Geometry: final body of the model. Coordinates: model frame, mm. Round coordinates to 2 decimals unless told otherwise and drop trailing zeros. Loops run counter-clockwise (first coordinate to the right, second up) from the corner with the lowest first, then second, coordinate; pieces in that order, holes last. Notation, with made-up numbers: M 5,29 L 58,29 A23 cw 58,40 Z; hole C 43.25,74.25 d3. An arc over 180 degrees is marked long. Answer as a JSON object with one key per item and string values.
from build123d import *

# Parameters (mm, degrees)
SKETCH1_R                   = 4.7625
BOSS_EXTRUDE1_DEPTH         = 12.7
FILLET1_R                   = 2.54
F_10_24_TAPPED_HOLE1_REACH  = 41.709
F_10_24_TAPPED_HOLE1_BORE_R = 1.89865


with BuildPart() as part:
    # Sketch1 → Boss-Extrude1 (new body)
    with BuildSketch(Plane.XY):
        with BuildLine():
            Line((-5.46431709, -20.393109008), (0, -11.1125))
            ThreePointArc((0, -11.1125), (11.017431022, -1.450472311), (2.876126639, 10.733850745))
            Line((2.876126639, 10.733850745), (0, 21.1125))
            ThreePointArc((0, 21.1125), (-20.931879636, 2.755734233), (-5.46431709, -20.393109008))
        make_face()
        Circle(SKETCH1_R, mode=Mode.SUBTRACT)
    extrude(amount=BOSS_EXTRUDE1_DEPTH)

    # Fillet1
    fillet1_edges = [part.edges().sort_by_distance(p)[0] for p in [
        (2.876126639, 10.733850745, 6.35),
        (0, -11.1125, 6.35),
        (-5.46431709, -20.393109008, 6.35),
        (0, 21.1125, 6.35),
    ]]
    fillet(fillet1_edges, radius=FILLET1_R)

    # #10-24 Tapped Hole1 bore (on position points) → #10-24 Tapped Hole1 (cut, up to next)
    with BuildSketch(Plane(origin=(11.019222387, -1.436799975, 6.35), x_dir=(0.129295835761, 0.99160606435, 0), z_dir=(0.99160606435, -0.129295835761, 0)), mode=Mode.PRIVATE) as f_10_24_tapped_hole1_sk1:
        with Locations((1e-09, 0)):
            Circle(F_10_24_TAPPED_HOLE1_BORE_R)
    f_10_24_tapped_hole1_tool1 = extrude(f_10_24_tapped_hole1_sk1.sketch, amount=-F_10_24_TAPPED_HOLE1_REACH, mode=Mode.PRIVATE) & part.part
    add(f_10_24_tapped_hole1_tool1.solids().sort_by_distance((11.019222, -1.4368, 6.35))[0], mode=Mode.SUBTRACT)


solid = part.part
1) Ray query, line 1 (Y direction, x = -1, z = 11.5); line 2 (X direction, y = 3.5, z = 4); line 3 (Y direction, x = 0, z = 9.75). Return the intervals inside material, ascending.
Results:
{"line 1": "-12.81 to -4.66, 4.66 to 20.85", "line 2": "-20.82 to -3.23, 3.23 to 10.55", "line 3": "-11.52 to -4.76, 4.76 to 20.15"}
2) Section query B-B (x = 0). Return the cut outline in (y, z).
Results:
{"outline": "M -11.52,0 L -4.76,0 L -4.76,12.7 L -11.52,12.7 Z; M 4.76,0 L 20.15,0 L 20.15,12.7 L 4.76,12.7 Z"}
3) Section query C-C (y = -1). Count the separate pieces of the cut face and the enclosed holes in it, and give its area (3 significant figures).
Results:
{"separate pieces": "3", "enclosed holes": "0", "area": "266 mm2"}
4) Section query D-D (x = -9). Return the cut outline in (y, z).
Results:
{"outline": "M -19.1,0 L 19.1,0 L 19.1,12.7 L -19.1,12.7 Z"}
5) Pull-direction query (Z, two-part tool) for faces 1 (the flat face through (-5, 1, 0)), 2 (the cylindrical face through (7.669, -1.415, 4.496)), 3 (the flat face through (-5, 1, 12.7)), 4 (the flat face through (-2.59, -15.51, 6.26)); classes: +Z half, -Z half, draft (parallel to the pull), parting line (faces both ways), or undercut.
Results:
{"face 1": "-Z half", "face 2": "undercut", "face 3": "+Z half", "face 4": "draft"}
6) Pin query (flat end, axial travel): P1, Ø1, axis at x = -2, y = -12.5, coming from the -Z side; P2, Ø2, axis at y = 17, z = 11, coming from the +X side; P3, Ø5, axis at y = 15, z = 6, coming from the -X side; P4, Ø1, axis at x = 0.5, z = 4.5, coming from the -Y side. Return the tip coordinate at first contact, or that it passes through.
Results:
{"P1": "z = 0", "P2": "x = 1.42", "P3": "x = -17.01", "P4": "y = -11.52"}
7) Section query A-A (z = 11.75). Return the cut outline in (x, y) (1 decimal).
Results:
{"outline": "M -7.5,-19.7 A2.5 ccw -4.4,-18.6 L -0.7,-12.3 A2.5 cw 1.2,-11 A11.1 ccw 4,10.4 A2.5 cw 2.5,12 L 0.5,19.2 A2.5 ccw -2.2,21 A21.1 ccw Z; hole C 0,0 d9.5"}
